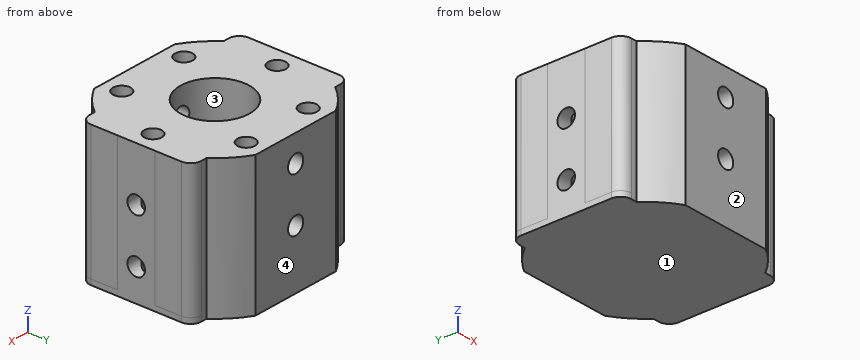
```python
from build123d import *
from build123d.topology import SkipClean

# Parameters (mm, degrees)
EXTRUDE_1_DEPTH      = 30
SKETCH_3_R           = 6.45
CUT_EXTRUDE_1_DEPTH  = 38.893765978
SKETCH_4_R           = 1.65
CUT_EXTRUDE_2_DEPTH  = 47.097722286
CUT_EXTRUDE_START    = -14
SKETCH_7_W           = 30
SKETCH_7_H           = 7
CUT_EXTRUDE_4_DEPTH  = 30
CUT_EXTRUDE_START_2  = 14
SKETCH_7_2_W         = 30
SKETCH_7_2_H         = 7
CUT_EXTRUDE_5_DEPTH  = 30
SKETCH_10_W          = 30
SKETCH_10_H          = 7
EXTRUDE_2_DEPTH      = 3.146428
SKETCH_11_W          = 30
SKETCH_11_H          = 7
EXTRUDE_3_DEPTH      = 3.146428
SKETCH_12_R          = 1.65
CUT_EXTRUDE_6_DEPTH  = 49.270720898
SKETCH_14_W          = 2.981852414
SKETCH_14_H          = 30.826717304
SKETCH_14_W_2        = 3.229128589
SKETCH_14_H_2        = 31.791094385
CUT_EXTRUDE_7_DEPTH  = 47.097722467
SKETCH_17_R          = 1.65
CUT_EXTRUDE_9_DEPTH  = 49.017575073
CUT_EXTRUDE_10_DEPTH = 5
SKETCH_19_R          = 1.65
CUT_EXTRUDE_11_DEPTH = 34.892292803
FILLET_1_R           = 2
EXTRUDE_START        = 1
EXTRUDE_6_DEPTH      = 1


with BuildPart() as part:
    # 草图1 → 凸台-拉伸1 (new body)
    with BuildSketch(Plane.XY):
        with BuildLine():
            Line((8.75, 15.155444566), (-8.75, 15.155444566))
            ThreePointArc((-8.75, 15.155444566), (-17.5, 0), (-8.75, -15.155444566))
            Line((-8.75, -15.155444566), (8.75, -15.155444566))
            ThreePointArc((8.75, -15.155444566), (17.5, 0), (8.75, 15.155444566))
        make_face()
    extrude(amount=EXTRUDE_1_DEPTH)

    # 草图3 → 切除-拉伸1 (cut, through all)
    with BuildSketch(Plane.XY.offset(30)):
        Circle(SKETCH_3_R)
    extrude(amount=-CUT_EXTRUDE_1_DEPTH, mode=Mode.SUBTRACT)

    # 草图4 → 切除-拉伸2 (cut, through all)
    with BuildSketch(Plane(origin=(0, 15.155444566, 0), x_dir=(1, 0, 0), z_dir=(0, 1, 0))):
        with Locations(Location((0, -15, 0), (0, 0, 180))):
            Circle(SKETCH_4_R)
        with Locations(Location((0, -25, 0), (0, 0, 180))):
            Circle(SKETCH_4_R)
    extrude(amount=-CUT_EXTRUDE_2_DEPTH, mode=Mode.SUBTRACT)

    # 草图7 → 切除-拉伸4 (cut)
    with BuildSketch(Plane(origin=(0, 0, 0), x_dir=(0, 0, -1), z_dir=(1, 0, 0)).offset(CUT_EXTRUDE_START)):
        with Locations((-15, 7)):
            Rectangle(SKETCH_7_W, SKETCH_7_H)
        with Locations((-15, -7)):
            Rectangle(SKETCH_7_W, SKETCH_7_H)
    extrude(amount=-CUT_EXTRUDE_4_DEPTH, mode=Mode.SUBTRACT)

    # 草图7<2> → 切除-拉伸5 (cut)
    with BuildSketch(Plane(origin=(0, 0, 0), x_dir=(0, 0, -1), z_dir=(1, 0, 0)).offset(CUT_EXTRUDE_START_2)):
        with Locations((-15, 7)):
            Rectangle(SKETCH_7_2_W, SKETCH_7_2_H)
        with Locations((-15, -7)):
            Rectangle(SKETCH_7_2_W, SKETCH_7_2_H)
    extrude(amount=CUT_EXTRUDE_5_DEPTH, mode=Mode.SUBTRACT)

    # 草图10 → 凸台-拉伸2 (add)
    with BuildSketch(Plane.ZY.offset(14)):
        with Locations((15, -7)):
            Rectangle(SKETCH_10_W, SKETCH_10_H)
        with Locations((15, 7)):
            Rectangle(SKETCH_10_W, SKETCH_10_H)
    extrude(amount=EXTRUDE_2_DEPTH)

    # 草图11 → 凸台-拉伸3 (add)
    with BuildSketch(Plane(origin=(14, 0, 0), x_dir=(0, 0, -1), z_dir=(1, 0, 0))):
        with Locations((-15, -7)):
            Rectangle(SKETCH_11_W, SKETCH_11_H)
        with Locations((-15, 7)):
            Rectangle(SKETCH_11_W, SKETCH_11_H)
    extrude(amount=EXTRUDE_3_DEPTH)

    # 草图12 → 切除-拉伸6 (cut, through all)
    with BuildSketch(Plane.ZY.offset(17.146428199)):
        with Locations((20, 0)):
            Circle(SKETCH_12_R)
    extrude(amount=-CUT_EXTRUDE_6_DEPTH, mode=Mode.SUBTRACT)

    # 草图14 → 切除-拉伸7 (cut, through all)
    with SkipClean():  # the faces are left unmerged after this step: merging them gives an invalid solid
        with BuildSketch(Plane.XZ.offset(15.155444566)):
            with Locations((-18.637354406, 14.586641348)):
                Rectangle(SKETCH_14_W, SKETCH_14_H)
            with Locations((18.760992494, 14.104452808)):
                Rectangle(SKETCH_14_W_2, SKETCH_14_H_2)
        extrude(amount=-CUT_EXTRUDE_7_DEPTH, mode=Mode.SUBTRACT)

    # 草图17 → 切除-拉伸9 (cut, through all)
    with SkipClean():  # the faces are left unmerged after this step: merging them gives an invalid solid
        with BuildSketch(Plane(origin=(17.146428199, 0, 0), x_dir=(0, 0, -1), z_dir=(1, 0, 0))):
            with Locations((-10, 0)):
                Circle(SKETCH_17_R)
        extrude(amount=-CUT_EXTRUDE_9_DEPTH, mode=Mode.SUBTRACT)

    # 草图18 → 切除-拉伸10 (cut)
    with BuildSketch(Plane(origin=(0, 0, 0), x_dir=(-1, 0, 0), z_dir=(0, 0, -1))):
        with BuildLine():
            Line((-14, 10.5), (-17.146428199, 10.5))
            Line((-17.146428199, 10.5), (-17.146428199, -10.5))
            Line((-17.146428199, -10.5), (-14, -10.5))
            ThreePointArc((-14, -10.5), (-11.610724182, -13.093551236), (-8.75, -15.155444566))
            Line((-8.75, -15.155444566), (8.75, -15.155444566))
            ThreePointArc((8.75, -15.155444566), (11.610724182, -13.093551236), (14, -10.5))
            Line((14, -10.5), (17.146428199, -10.5))
            Line((17.146428199, -10.5), (17.146428199, 10.5))
            Line((17.146428199, 10.5), (14, 10.5))
            ThreePointArc((14, 10.5), (11.610724182, 13.093551236), (8.75, 15.155444566))
            Line((8.75, 15.155444566), (-8.75, 15.155444566))
            ThreePointArc((-8.75, 15.155444566), (-11.610724182, 13.093551236), (-14, 10.5))
        make_face()
    extrude(amount=-CUT_EXTRUDE_10_DEPTH, mode=Mode.SUBTRACT)

    # 草图19 → 切除-拉伸11 (cut, through all)
    with BuildSketch(Plane.XY.offset(30)):
        with Locations((13.5, 0)):
            Circle(SKETCH_19_R)
        with Locations((6.75, -11.691342951)):
            Circle(SKETCH_19_R)
        with Locations((-6.75, -11.691342951)):
            Circle(SKETCH_19_R)
        with Locations((-13.5, 0)):
            Circle(SKETCH_19_R)
        with Locations((-6.75, 11.691342951)):
            Circle(SKETCH_19_R)
        with Locations((6.75, 11.691342951)):
            Circle(SKETCH_19_R)
    extrude(amount=-CUT_EXTRUDE_11_DEPTH, mode=Mode.SUBTRACT)

    # 圆角1
    fillet_1_edges = [part.edges().sort_by_distance(p)[0] for p in [
        (-17.146428, 10.5, 17.5),
        (17.146428, -10.5, 17.5),
        (17.146428, 10.5, 17.5),
        (-17.146428, -10.5, 17.5),
    ]]
    fillet(fillet_1_edges, radius=FILLET_1_R)

    # 草图24 → 凸台-拉伸6 (add)
    with BuildSketch(Plane(origin=(0, 0, 5), x_dir=(-1, 0, 0), z_dir=(0, 0, -1)).offset(EXTRUDE_START)):
        with BuildLine():
            Line((-17.146428199, 8.5), (-17.146428199, -8.5))
            ThreePointArc((-17.146428199, -8.5), (-16.560641762, -9.914213562), (-15.146428199, -10.5))
            Line((-15.146428199, -10.5), (-14, -10.5))
            ThreePointArc((-14, -10.5), (-11.610724182, -13.093551236), (-8.75, -15.155444566))
            Line((-8.75, -15.155444566), (8.75, -15.155444566))
            ThreePointArc((8.75, -15.155444566), (11.610724182, -13.093551236), (14, -10.5))
            Line((14, -10.5), (15.146428199, -10.5))
            ThreePointArc((15.146428199, -10.5), (16.560641762, -9.914213562), (17.146428199, -8.5))
            Line((17.146428199, -8.5), (17.146428199, 8.5))
            ThreePointArc((17.146428199, 8.5), (16.560641762, 9.914213562), (15.146428199, 10.5))
            Line((15.146428199, 10.5), (14, 10.5))
            ThreePointArc((14, 10.5), (11.610724182, 13.093551236), (8.75, 15.155444566))
            Line((8.75, 15.155444566), (-8.75, 15.155444566))
            ThreePointArc((-8.75, 15.155444566), (-11.610724182, 13.093551236), (-14, 10.5))
            Line((-14, 10.5), (-15.146428199, 10.5))
            ThreePointArc((-15.146428199, 10.5), (-16.560641762, 9.914213562), (-17.146428199, 8.5))
        make_face()
    extrude(amount=-EXTRUDE_6_DEPTH)


solid = part.part
```
Verification items for the finished model (mm, model axes). Face numbers are marked on the shaded views. Give positions to 0.01 mm unless a question says otherwise; leave off trailing zeros. Write each loop counter-clockwise with the first axis right and the second up, starting at its lowest first coordinate (ties: lowest second). Pieces come first, ordered by that corner, then holes. Notation, with made-up numbers: (-40, -1.75) - (-28, -1.75) arc R17 ccw to (-28, 23.25) - close; hole circle Ø3 at (6.5, -16.75). An arc over 180 degrees is marked (long way). Put each result on its own line as item: value.
Q1. Scan lines: probe 1 along X at (y, z) = (0, 26.25); probe 2 along Y at (x, z) = (6.75, 25); probe 3 along X at (y, z) = (-12, 22.25). Record each from-to range of solid material in increasing order. Write a range as from..to.
Result:
probe 1: -17.15..-15.15, -11.85..-6.45, 6.45..11.85, 15.15..17.15
probe 2: -15.16..-13.34, -10.04..10.04, 13.34..15.16
probe 3: -12.74..-8.37, -5.13..5.13, 8.37..12.74
Q2. Section check C-C on y = 0. Count the separate pieces of the cut face and the enclosed holes in it, and give its area (3 significant figures).
Result:
separate pieces: 9
enclosed holes: 0
area: 306 mm2
Q3. Mould release check, pull along Y, two halves, no side actions. Record for the marked faces 1, 2, 3 and 4: released by +Y, released by -Y, zero draft, split by the parting line, or undercut.
Result:
face 1: zero draft
face 2: released by -Y
face 3: undercut
face 4: released by +Y
Q4. Section check B-B on x = 1. Record the cut outline in (y, z), and give its area (3 significant figures).
Result:
outline: (-15.16, 4) - (15.16, 4) - (15.16, 13.69) - (6.37, 13.69) - (6.37, 5) - (-6.37, 5) - (-6.37, 13.69) - (-15.16, 13.69) - close; (-15.16, 16.31) - (-6.37, 16.31) - (-6.37, 23.69) - (-15.16, 23.69) - close; (-15.16, 26.31) - (-6.37, 26.31) - (-6.37, 30) - (-15.16, 30) - close; (6.37, 16.31) - (15.16, 16.31) - (15.16, 23.69) - (6.37, 23.69) - close; (6.37, 26.31) - (15.16, 26.31) - (15.16, 30) - (6.37, 30) - close
area: 377 mm2
Q5. Section check A-A on z = 12.75. Record the cut outline in (x, y).
Result:
outline: (-17.15, -8.5) arc R2 ccw to (-15.15, -10.5) - (-14, -10.5) arc R17.5 ccw to (-8.75, -15.16) - (8.75, -15.16) arc R17.5 ccw to (14, -10.5) - (15.15, -10.5) arc R2 ccw to (17.15, -8.5) - (17.15, 8.5) arc R2 ccw to (15.15, 10.5) - (14, 10.5) arc R17.5 ccw to (8.75, 15.16) - (-8.75, 15.16) arc R17.5 ccw to (-14, 10.5) - (-15.15, 10.5) arc R2 ccw to (-17.15, 8.5) - close; hole circle Ø3.3 at (-13.5, 0); hole circle Ø3.3 at (-6.75, -11.69); hole circle Ø3.3 at (-6.75, 11.69); hole circle Ø12.9 at (0, 0); hole circle Ø3.3 at (6.75, -11.69); hole circle Ø3.3 at (6.75, 11.69); hole circle Ø3.3 at (13.5, 0)
Q6. Depth check by flat-ended pin: P1, Ø2, axis at x = 0, z = 15, coming from the -Y side; P2, Ø1.7, axis at x = 7.5, y = -12.5, coming from the +Z side; P3, Ø2, axis at x = -6.75, y = 11.69, coming from the +Z side. Enter the tip coordinate at first touch or a pass-through.
Result:
P1: through
P2: z = 30
P3: z = 5
